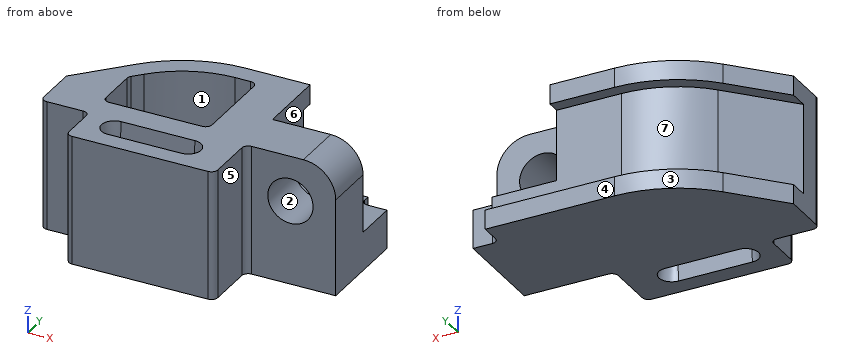
```python
from build123d import *

# Parameters (mm, degrees)
BOSS_EXTRUDE1_DEPTH     = 50
CUT_EXTRUDE1_DEPTH      = 231.236834586
CUT_EXTRUDE1_DEPTH_BACK = 85
SKETCH3_W               = 70
SKETCH3_H               = 70
CUT_EXTRUDE2_DEPTH      = 55
SKETCH4_R               = 17.5
CUT_EXTRUDE3_DEPTH      = 183.027470454
CUT_EXTRUDE4_DEPTH      = 35
FILLET1_R               = 5
FILLET2_R               = 5
CUT_EXTRUDE5_DEPTH      = 25
CUT_EXTRUDE5_DRAFT      = -5
MIRROR1_COPY_1_DEPTH    = 25
MIRROR1_COPY_1_DRAFT    = -5


with BuildPart() as part:
    # Sketch1 → Boss-Extrude1 (new, symmetric)
    with BuildSketch(Plane.XY):
        with BuildLine():
            Line((0, 0), (-115, 0))
            Line((-115, 0), (-115, 35))
            Line((-115, 35), (-153, 35))
            Line((-153, 35), (-153, 73))
            Line((-153, 73), (-118.15707843, 110.364458857))
            ThreePointArc((-118.15707843, 110.364458857), (-87.160639926, 132.270575779), (-50, 140))
            Line((-50, 140), (50, 140))
            Line((50, 140), (50, 120))
            Line((50, 120), (70, 120))
            Line((70, 120), (70, 45))
            Line((70, 45), (0, 45))
            Line((0, 45), (0, 0))
        make_face()
    extrude(amount=BOSS_EXTRUDE1_DEPTH, both=True)

    # Sketch2 → Cut-Extrude1 (cut, two sides: drawn at the far end of the back side and taken through both)
    with BuildSketch(Plane.XY.offset(50).offset(-CUT_EXTRUDE1_DEPTH_BACK)):
        with BuildLine():
            Line((-33, 54), (-33, 125))
            Line((-33, 125), (-50, 125))
            ThreePointArc((-50, 125), (-81.179403892, 118.514674664), (-107.186772906, 100.134483456))
            Line((-107.186772906, 100.134483456), (-115, 91.755823196))
            Line((-115, 91.755823196), (-115, 54))
            Line((-115, 54), (-33, 54))
        make_face()
    extrude(amount=CUT_EXTRUDE1_DEPTH + CUT_EXTRUDE1_DEPTH_BACK, mode=Mode.SUBTRACT)

    # Sketch3 → Cut-Extrude2 (cut)
    with BuildSketch(Plane(origin=(0, 140, 0), x_dir=(1, 0, 0), z_dir=(0, 1, 0))):
        with Locations((35, -15)):
            Rectangle(SKETCH3_W, SKETCH3_H)
    extrude(amount=-CUT_EXTRUDE2_DEPTH, mode=Mode.SUBTRACT)

    # Sketch4 → Cut-Extrude3 (cut, through all)
    with BuildSketch(Plane(origin=(0, 85, 0), x_dir=(1, 0, 0), z_dir=(0, 1, 0))):
        with Locations(Location((35, -15, 0), (0, 0, 180))):
            Circle(SKETCH4_R)
        with BuildLine():
            Line((70, -25), (70, -50))
            Line((70, -50), (45, -50))
            ThreePointArc((45, -50), (62.67766953, -42.67766953), (70, -25))
        make_face()
    extrude(amount=-CUT_EXTRUDE3_DEPTH, mode=Mode.SUBTRACT)

    # Sketch5 → Cut-Extrude4 (cut, symmetric)
    with BuildSketch(Plane.XY):
        with BuildLine():
            Line((-110.843541414, 103.544475257), (-153, 58.337208144))
            Line((-153, 58.337208144), (-153, 73))
            Line((-153, 73), (-118.15707843, 110.364458857))
            ThreePointArc((-118.15707843, 110.364458857), (-87.160639926, 132.270575779), (-50, 140))
            Line((-50, 140), (0, 140))
            Line((0, 140), (50, 140))
            Line((50, 140), (50, 130))
            Line((50, 130), (0, 130))
            Line((0, 130), (-50, 130))
            ThreePointArc((-50, 130), (-83.173149237, 123.099975036), (-110.843541414, 103.544475257))
        make_face()
    extrude(amount=CUT_EXTRUDE4_DEPTH, both=True, mode=Mode.SUBTRACT)

    # Fillet1
    fillet1_edges = [part.edges().sort_by_distance(p)[0] for p in [
        (-115, 91.755823196, 7.5),
        (-33, 125, 7.5),
        (-33, 54, 7.5),
        (-115, 54, 7.5),
    ]]
    fillet(fillet1_edges, radius=FILLET1_R)

    # Fillet2
    fillet2_edges = [part.edges().sort_by_distance(p)[0] for p in [
        (0, 0, 0),
        (-115, 0, 0),
        (-115, 35, 0),
        (-153, 35, 0),
        (0, 45, 0),
        (50, 120, -35),
    ]]
    fillet(fillet2_edges, radius=FILLET2_R)


with BuildPart() as cut_extrude5_tool:
    # Sketch6 → Cut-Extrude5 (with draft: the straight prism first)
    with BuildSketch(Plane.XY.offset(50)):
        with BuildLine():
            ThreePointArc((-90, 34), (-100, 24), (-90, 14))
            Line((-90, 14), (-33, 14))
            ThreePointArc((-33, 14), (-23, 24), (-33, 34))
            Line((-33, 34), (-90, 34))
        make_face()
    extrude(amount=-CUT_EXTRUDE5_DEPTH)
    # Cut-Extrude5: the draft: its side faces are tilted about the plane it starts from
    cut_extrude5_sides = [cut_extrude5_tool.faces().sort_by_distance(p)[0] for p in [
        (-23, 24, 37.5),
        (-61.5, 34, 37.5),
        (-100, 24, 37.5),
        (-61.5, 14, 37.5),
    ]]
    draft(cut_extrude5_sides, Plane.XY.offset(50), CUT_EXTRUDE5_DRAFT)


with BuildPart() as part_1:
    add(part.part)

    # Cut-Extrude5: cut by cut_extrude5_tool
    add(cut_extrude5_tool.part, mode=Mode.SUBTRACT)


with BuildPart() as mirror1_copy_1_tool:
    # Mirror1 copy 1 sketch → Mirror1 copy 1 (with draft: the straight prism first)
    with BuildSketch(Plane(origin=(0, 0, -50), x_dir=(1, 0, 0), z_dir=(0, 0, -1))):
        with BuildLine():
            ThreePointArc((-90, -34), (-100, -24), (-90, -14))
            Line((-90, -14), (-33, -14))
            ThreePointArc((-33, -14), (-23, -24), (-33, -34))
            Line((-33, -34), (-90, -34))
        make_face()
    extrude(amount=-MIRROR1_COPY_1_DEPTH)
    # Mirror1 copy 1: the draft: its side faces are tilted about the plane it starts from
    mirror1_copy_1_sides = [mirror1_copy_1_tool.faces().sort_by_distance(p)[0] for p in [
        (-23, 24, -37.5),
        (-61.5, 34, -37.5),
        (-100, 24, -37.5),
        (-61.5, 14, -37.5),
    ]]
    draft(mirror1_copy_1_sides, Plane(origin=(0, 0, -50), x_dir=(1, 0, 0), z_dir=(0, 0, -1)), MIRROR1_COPY_1_DRAFT)


with BuildPart() as part_2:
    add(part_1.part)

    # Mirror1 copy 1: cut by mirror1_copy_1_tool
    add(mirror1_copy_1_tool.part, mode=Mode.SUBTRACT)


solid = part_2.part
```
Verification items for the finished model (mm, model axes). Face numbers are marked on the shaded views. A direction names the side the tool comes from. Give positions to 0.01 mm unless a question says otherwise; leave off trailing zeros. Loops run counter-clockwise (first coordinate to the right, second up) from the corner with the lowest first, then second, coordinate; pieces in that order, holes last. Notation, with made-up numbers: M -20.5,75 L -0.5,75 A26 cw -0.5,98 Z; hole C 18.5,86 d11. An arc over 180 degrees is marked long. One line per question, with ' | ' between items.
Item 1: Section check A-A, the plane z = 15. State how many separate pieces and enclosed holes the cut face has, plus the area to 3 significant figures.
Completed:
separate pieces: 2 | enclosed holes: 1 | area: 12,300 mm^2
Item 2: Draft check along X on the marked faces 1, 2, 3 and 4. Enter one of: +X half, -X half, draft (parallel to the pull), parting line (faces both ways), or undercut.
Completed:
face 1: undercut | face 2: undercut | face 3: -X half | face 4: draft
Item 3: Section check B-B, the plane x = 35. Record the cut outline in (y, z), plus the area to 3 significant figures.
Completed:
outline: M 45,-50 L 140,-50 L 140,-35 L 130,-35 L 130,-20 L 85,-20 L 85,-2.5 L 45,-2.5 Z; M 45,32.5 L 85,32.5 L 85,50 L 45,50 Z | area: 4,100 mm^2
Item 4: Section check D-D, the plane z = -40. Record the cut outline in (x, y), plus the area to 3 significant figures.
Completed:
outline: M -153,40 A5 ccw -148,35 L -120,35 A5 cw -115,30 L -115,5 A5 ccw -110,0 L -5,0 A5 ccw 0,5 L 0,40 A5 cw 5,45 L 70,45 L 70,120 L 55,120 A5 cw 50,125 L 50,140 L -50,140 A93.19 ccw -118.16,110.36 L -153,73 Z; hole M -90,14.87 L -33,14.87 A9.13 ccw -33,33.13 L -90,33.13 A9.13 ccw Z | area: 22,700 mm^2
Item 5: Tool access check on the marked faces 5, 6 and 7. Record the directions out of +Z, -Z, +X, -X, +Y, -Y that give a thin tool (end or side, any length) a straight path to the whole face; none if there is none.
Completed:
face 5: +Z, -Z, +X, -Y | face 6: +Z, +X, +Y | face 7: -X, +Y
Item 6: Depth check by flat-ended pin: P1, Ø1.5, axis at y = 64, z = -32.5, coming from the -X side; P2, Ø1.5, axis at y = 124.5, z = 21.5, coming from the +X side; P3, Ø16.5, axis at x = 63, z = -40, coming from the +Y side. Enter the tip coordinate at first touch or a pass-through.
Completed:
P1: stops at x = -148.42 | P2: stops at x = 0 | P3: stops at y = 120.01
Item 7: Section check C-C, the plane y = 24. Record the cut outline in (x, z), plus the area to 3 significant figures.
Completed:
outline: M -115,-50 L -100,-50 L -97.81,-25 L -25.19,-25 L -23,-50 L 0,-50 L 0,50 L -23,50 L -25.19,25 L -97.81,25 L -100,50 L -115,50 Z | area: 7,760 mm^2
Item 8: Thickness scan on line 1 (Z direction, x = 35, y = 69); line 2 (X direction, y = 81, z = 28); line 3 (Y direction, x = -44.5, z = -38). Record the ranges inside material, lowest first. Write a range as [from, to].
Completed:
line 1: z = [-50, -2.5], [32.5, 50] | line 2: x = [-131.87, -115], [-33, 23.28], [46.72, 69.82] | line 3: y = [0, 15.05], [32.95, 140]
